The model under review builds one solid part; all positions refer to its coordinate system, in mm. A direction names the side the tool comes from. Give positions to 0.01 mm unless a question says otherwise; leave off trailing zeros. Order: outer loops, then holes, each group sorted by start corner. A loop starts at its lowest first (then second) coordinate and runs counter-clockwise, first axis right, second up. Notation, with made-up numbers: (35, -26.5) -> (90, -26.5) arc R30 cw to (90, 7.5) -> close; hole circle Ø5 at (52, 61). An arc over 180 degrees is marked (long way). Answer as a JSON object with one key per item and string values. Group by question number.
from build123d import *

# Parameters (mm, degrees)
F1_DEPTH = 35.56
F2_W     = 10.16
F2_H     = 50.038
F3_DEPTH = 71.121
F4_R     = 19.356185
F5_DEPTH = 67.173316


with BuildPart() as f1:
    # F0 (on Front) → F1 (new body, symmetric)
    with BuildSketch(Plane.XZ):
        Polygon((-35.56, 41.656), (-35.56, 0), (35.56, 0), (35.56, 23.876), (-2.54, 61.976), (-15.24, 61.976), align=None)
    extrude(amount=F1_DEPTH, both=True)

    # F2 (on face) → F3 (cut, through all)
    with BuildSketch(Plane.YZ.offset(35.56)):
        with Locations((-30.48, 36.957)):
            Rectangle(F2_W, F2_H)
        with Locations((30.48, 36.957)):
            Rectangle(F2_W, F2_H)
    extrude(amount=-F3_DEPTH, mode=Mode.SUBTRACT)

    # F4 (on face) → F5 (cut, through all)
    with BuildSketch(Plane(origin=(29.718, 0, 29.718), x_dir=(0.707107, 0, -0.707107), z_dir=(0.707107, 0, 0.707107))):
        with Locations((-18.183183, 0)):
            Circle(F4_R)
    extrude(amount=-F5_DEPTH, mode=Mode.SUBTRACT)


solid = f1.part
1. For probe 1 along Y at (x, z) = (-18.5, 8.5); probe 2 along Z at (x, y) = (-30.5, -29); probe 3 along Y at (x, z) = (18.5, 36), list the stretches that pass through material, from the lowest coordinate up. Write a range as [from, to].
2. Machinability: for faces 4 (the flat face through (-25.258, -0.356, 51.958)), 5 (the flat face through (0, -31, 11.938)), 6 (the flat face through (0, 30, 11.938)), which of the approach directions +Z, -Z, +X, -X, +Y, -Y give a long, thin tool a straight path to every point of the face, cutting with its end or side? Answer none if there is none.
3. For pin 1 (11 mm diameter, centred on x = -17, y = 32, fed in from +Z); pin 2 (1 mm diameter, centred on y = -27.5, z = 36, fed in from +X); pin 3 (25 mm diameter, centred on x = 0, z = 29, fed in from +Y); pin 4 (6 mm diameter, centred on y = 28, z = 46, fed in from -X), all flat-tipped, find the tip position at first contact; note any pin that passes through.
4. Take a section at A-A on y = 6.5. Give the boundary of the cut face in (x, z), plus the area to 3 significant figures.
5. Draft analysis for pull direction Y (two halves, no side actions). For faces 1 (the flat face through (-9, 0, 61.976)), 2 (the cylindrical face through (-14.95, 0.85, 38.11)), 3 (the flat face through (-7, -25.4, 31)), state which applies: pulls with the +Y half, pulls with the -Y half, needs draft (parallel to the pull), parting line crosses it, or undercut.
6. Take a section at B-B on y = -1. Give the boundary of the cut face in (x, z).
7. Take a section at C-C on y = 27. Give the boundary of the cut face in (x, z).
Checks:
{
 "1": {"probe 1": "y = [-35.56, -19.33], [19.33, 35.56]", "probe 2": "z = [0, 11.94]", "probe 3": "y = [-25.4, -18.46], [18.46, 25.4]"},
 "2": {"face 4": "+Z, -X, +Y, -Y", "face 5": "+Z, +X, -X, -Y", "face 6": "+Z, +X, -X, +Y"},
 "3": {"pin 1": "stops at z = 11.94", "pin 2": "passes through", "pin 3": "stops at y = 25.4", "pin 4": "stops at x = -32.71"},
 "4": {"outline": "(-35.56, 15.94) -> (3.97, 55.47) -> (-2.54, 61.98) -> (-15.24, 61.98) -> (-35.56, 41.66) -> close; (0.07, 0) -> (35.56, 0) -> (35.56, 23.88) -> (29.75, 29.68) -> close", "area": "1,410 mm2"},
 "5": {"face 1": "needs draft", "face 2": "undercut", "face 3": "pulls with the -Y half"},
 "6": {"outline": "(-35.56, 17.49) -> (3.19, 56.24) -> (-2.54, 61.98) -> (-15.24, 61.98) -> (-35.56, 41.66) -> close; (1.62, 0) -> (35.56, 0) -> (35.56, 23.88) -> (30.53, 28.91) -> close"},
 "7": {"outline": "(-35.56, 0) -> (35.56, 0) -> (35.56, 11.94) -> (-35.56, 11.94) -> close"}
}
